Read the model definition and answer for the solid it produces. Units are mm, in the model's axes. A direction names the side the tool comes from. Round coordinates to 2 decimals unless told otherwise and drop trailing zeros. Loops run counter-clockwise (first coordinate to the right, second up) from the corner with the lowest first, then second, coordinate; pieces in that order, holes last. Notation, with made-up numbers: (15.5, 4) - (60.5, 4) arc R37 ccw to (60.5, 42) - close; hole circle Ø6 at (-12, 69). An arc over 180 degrees is marked (long way). Answer as CSV lines item,"result".
Autodesk Inventor part; units mm, degrees
ref_plane "YZ Plane" through (0, 0, 0) normal (1, 0, 0) x (0, 1, 0)
ref_plane "XZ Plane" through (0, 0, 0) normal (0, 1, 0) x (-1, 0, 0)
ref_plane "XY Plane" through (0, 0, 0) normal (0, 0, 1) x (1, 0, 0)
sketch "Sketch1" plane through (0, 0, 0) normal (0, 0, 1) x (1, 0, 0)
  circle A0 centre (4, 4) radius 1.2
  circle A1 centre (4, 4) radius 2
  point P0 (0, 0)
  dimension "d0" = 4
extrude "Extrusion1" add sketch "Sketch1" against normal blind 20 contours A0 | A1
sketch "Sketch2" plane through (4, 4, 0) normal (0, 0, 1) x (1, 0, 0)
  circle A0 centre (0, 0) radius 2
  circle A1 centre (0, 0) radius 3.65
  point P0 (-4, -4)
  dimension "d3" = 7.3
extrude "Extrusion2" add sketch "Sketch2" along normal blind 2.3 contours A0 | A1
fillet "Fillet1" radius 2.2 1 edges at (0.35, 4, 2.3)
sketch "Sketch4" plane through (4, 4, 2.3) normal (0, 0, 1) x (1, 0, 0)
  circle A0 centre (0, 0) radius 1.45
  line L0 (0.7217, 1.25) -> (1.4434, 0)
  line L1 (1.4434, 0) -> (0.7217, -1.25)
  line L2 (0.7217, -1.25) -> (-0.7217, -1.25)
  line L3 (-0.7217, -1.25) -> (-1.4434, 0)
  line L4 (-1.4434, 0) -> (-0.7217, 1.25)
  line L5 (-0.7217, 1.25) -> (0.7217, 1.25)
  point P0 (-4, -4)
  dimension "d10" = 2.5
extrude "Extrusion4" cut sketch "Sketch4" along normal mid plane 4 contours L0 L1 L2 L3 L4 L5
thread "Thread1"
properties part number "m3 6" material "Steel"
1) A cutting plane is placed at A-A, the plane z = -10.75. Determine the outline of the cut face in (x, y), plus the area to 3 significant figures.
Entries:
outline,"circle Ø4 at (4, 4)"
area,"12.6 mm^2"
2) Find the intervals of material crossed by line 1 (Z direction, x = 5.5, y = 3.5); line 2 (Y direction, x = 4, z = -18.25); line 3 (X direction, y = 3, z = 1.25), in increasing order.
Entries:
line 1,"z = -20 to 2.3"
line 2,"y = 2 to 6"
line 3,"x = 0.83 to 3.13, 4.87 to 7.17"
3) The mould has two halves that part along Y. Classify faces 1 (the face through (2.4, 2.8, -9.9)), 2 (the face through (2.912, 4.616, 1.286)), 3 (the face through (6, 2, 0)): pulls with the +Y half, pulls with the -Y half, needs draft (parallel to the pull), parting line crosses it, or undercut.
Entries:
face 1,"parting line crosses it"
face 2,"undercut"
face 3,"needs draft"
4) Each of these flat-tipped pins is pushed along its axis until it touches: P1, Ø1.2, axis at x = 3.5, z = 1.5, coming from the +Y side; P2, Ø1, axis at x = 2.5, y = 1.5, coming from the -Z side; P3, Ø1.6, axis at x = 4, z = 1, coming from the -Y side. Where does it stop, or does it pass through?
Entries:
P1,"stops at y = 7.47"
P2,"stops at z = 0"
P3,"stops at y = 0.35"
5) A tool of negligible diameter and unlimited length cuts with its end or side. For faces 4 (the face through (5.08, 4.63, 1.29)), 5 (the face through (4, 4, -20)), from which of +Z, -Z, +X, -X, +Y, -Y can it reach the whole face along a straight path? Write none if from no direction.
Entries:
face 4,"+Z"
face 5,"-Z, +X, -X, +Y, -Y"
